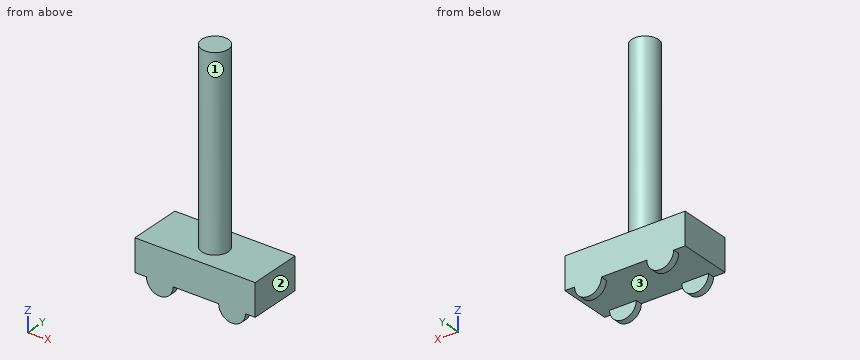
```python
from build123d import *

# Parameters (mm, degrees)
F0_W     = 114.3
F0_H     = 50.8
F1_DEPTH = 30.48
F2_R     = 12.7
F3_DEPTH = 177.8
F5_DEPTH = 6.35
F7_DEPTH = 6.35


with BuildPart() as f1:
    # F0 (on Top) → F1 (new body)
    with BuildSketch(Plane.XY):
        Rectangle(F0_W, F0_H)
    extrude(amount=F1_DEPTH)

    # F2 (on face) → F3 (join)
    with BuildSketch(Plane.XY.offset(30.48)):
        Circle(F2_R)
    extrude(amount=F3_DEPTH)

    # F4 (on face) → F5 (join)
    with BuildSketch(Plane(origin=(0, 25.4, 0), x_dir=(-1, 0, 0), z_dir=(0, 1, 0))):
        with BuildLine():
            Line((-47.841646862, 0), (-22.441646862, 0))
            ThreePointArc((-22.441646862, 0), (-35.141646862, 12.7), (-47.841646862, 0))
        make_face()
        with BuildLine():
            ThreePointArc((-47.841646862, 0), (-35.141646862, -12.7), (-22.441646862, 0))
            Line((-22.441646862, 0), (-47.841646862, 0))
        make_face()
        with BuildLine():
            Line((46.138353138, 0), (20.738353138, 0))
            ThreePointArc((20.738353138, 0), (33.438353138, -12.7), (46.138353138, 0))
        make_face()
    extrude(amount=-F5_DEPTH)

    # F6 (on face) → F7 (join)
    with BuildSketch(Plane.XZ.offset(25.4)):
        with BuildLine():
            ThreePointArc((-46.1274172783, 0), (-33.4274172783, -12.7), (-20.7274172783, 0))
            Line((-20.7274172783, 0), (-46.1274172783, 0))
        make_face()
        with BuildLine():
            Line((47.8525827217, 0), (22.4525827217, 0))
            ThreePointArc((22.4525827217, 0), (35.1525827217, -12.7), (47.8525827217, 0))
        make_face()
        with BuildLine():
            ThreePointArc((47.8525827217, 0), (35.1525827217, 12.7), (22.4525827217, 0))
            Line((22.4525827217, 0), (47.8525827217, 0))
        make_face()
    extrude(amount=-F7_DEPTH)


solid = f1.part
```
The model under review builds one solid part; all positions refer to its coordinate system, in mm. Face numbers are marked on the shaded views. Round coordinates to 2 decimals unless told otherwise and drop trailing zeros. Write each loop counter-clockwise with the first axis right and the second up, starting at its lowest first coordinate (ties: lowest second). Pieces come first, ordered by that corner, then holes. Notation, with made-up numbers: (12, 4.5) - (53, 4.5) arc R15 cw to (53, 31.5) - close; hole circle Ø6 at (-28.75, 58.25). An arc over 180 degrees is marked (long way). Answer as CSV lines item,"result". Start each with the question number.
(1) We need section A-A on x = 0. State the section outline as (y, z) points, plus the area to 3 significant figures.
(2) For pin 1 Ø5 at (y, z) = (7.5, 82) entering from +X; pin 2 Ø10 at (y, z) = (-7.5, 62.5) entering from +X; pin 3 Ø6 at (x, y) = (35, -13.5) entering from -Z; pin 4 Ø12 at (x, z) = (19.5, 40) entering from -Y, all flat-tipped, find the tip position at first contact; note any pin that passes through.
(3) To check wall thickness, follow line 1 (Z direction, x = 8.5, y = 14.5); line 2 (Z direction, x = -1.5, y = -7.5); line 3 (X direction, y = 0.5, z = 144). State the ranges of each line that lie inside material, in increasing order.
(4) Draft analysis for pull direction Y (two halves, no side actions). For the marked faces 1, 2 and 3, state which applies: pulls with the +Y half, pulls with the -Y half, needs draft (parallel to the pull), parting line crosses it, or undercut.
(5) We need section C-C on z = 79. State the section outline as (x, y) points.
(6) We need section B-B on y = 0. State the section outline as (x, z) points.
(7) We need section D-D on x = -18.5. State the section outline as (y, z) points.
Worked answers:
1,outline,"(-25.4, 0) - (25.4, 0) - (25.4, 30.48) - (12.7, 30.48) - (12.7, 208.28) - (-12.7, 208.28) - (-12.7, 30.48) - (-25.4, 30.48) - close"
1,area,"6,060 mm²"
2,pin 1,"x = 11.67"
2,pin 2,"x = 12.45"
2,pin 3,"z = 0"
2,pin 4,"through"
3,line 1,"0 to 30.48"
3,line 2,"0 to 208.28"
3,line 3,"-12.69 to 12.69"
4,face 1,"parting line crosses it"
4,face 2,"needs draft"
4,face 3,"undercut"
5,outline,"circle Ø25.4 at (0, 0)"
6,outline,"(-57.15, 0) - (57.15, 0) - (57.15, 30.48) - (12.7, 30.48) - (12.7, 208.28) - (-12.7, 208.28) - (-12.7, 30.48) - (-57.15, 30.48) - close"
7,outline,"(-25.4, 0) - (25.4, 0) - (25.4, 30.48) - (-25.4, 30.48) - close"
